from build123d import *

# Parameters (mm, degrees)
F0_W     = 231
F0_H     = 310
F1_DEPTH = 4
F2_W     = 310
F2_H     = 16
F3_DEPTH = 4


with BuildPart() as f1:
    # F0 (on Top) → F1 (new body)
    with BuildSketch(Plane.XY):
        with Locations((115.5, 155)):
            Rectangle(F0_W, F0_H)
    extrude(amount=F1_DEPTH)

    # F2 (on Right) → F3 (join)
    with BuildSketch(Plane.YZ):
        with Locations((155, 8)):
            Rectangle(F2_W, F2_H)
    extrude(amount=F3_DEPTH)

    # F4: F1 across face


with BuildPart() as f1_1:
    add(f1.part)
    add(f1.part.mirror(Plane(origin=(231, 155, 2), x_dir=(0, 1, 0), z_dir=(1, 0, 0))))

    # F5: F1 across face


with BuildPart() as f1_2:
    add(f1_1.part)
    add(f1_1.part.mirror(Plane(origin=(231, 0, 2.395062), x_dir=(1, 0, 0), z_dir=(0, -1, 0))))


solid = f1_2.part
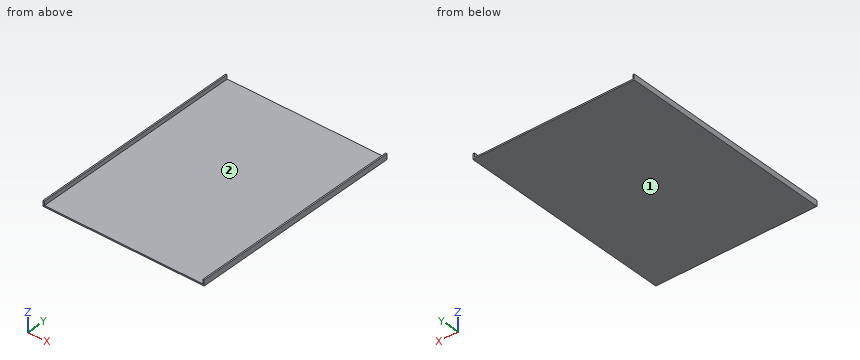
Input: part model. Units: mm. Frame: model coordinates. Face numbers are marked on the shaded views. Coordinates: 2 decimals unless noted, no trailing zeros. Loops run counter-clockwise (first coordinate to the right, second up) from the corner with the lowest first, then second, coordinate; pieces in that order, holes last. Notation, with made-up numbers: (-39.75, 68) -> (-5.75, 68) arc R9 ccw to (-5.75, 80) -> close; hole circle Ø7 at (-4, 17). An arc over 180 degrees is marked (long way). Write each question's results on one line, items separated by ' | '. Start each with the question number.
Q1. Section C-C, the plane x = 307. Return the cut outline in (y, z), plus the area to 3 significant figures.
Q2. Section B-B, the plane y = -42.5. Return the cut outline in (x, z), plus the area to 3 significant figures.
Q3. Pull-direction query (X, two-part tool) for the marked faces 1 and 2; classes: released by +X, released by -X, zero draft, split by the parting line, or undercut.
Q4. Section A-A, the plane z = 11. Return the cut outline in (x, y).
Q5. Ray query, line 1 (X direction, y = -243.5, z = 9.5); line 2 (Z direction, x = 177.5, y = 120). Return the intervals inside material, ascending. Write a range as from..to.
Found:
1) outline: (-310, 0) -> (310, 0) -> (310, 4) -> (-310, 4) -> close | area: 2,480 mm2
2) outline: (0, 0) -> (462, 0) -> (462, 16) -> (458, 16) -> (458, 4) -> (4, 4) -> (4, 16) -> (0, 16) -> close | area: 1,940 mm2
3) face 1: zero draft | face 2: undercut
4) outline: (0, -310) -> (4, -310) -> (4, 310) -> (0, 310) -> close; (458, -310) -> (462, -310) -> (462, 310) -> (458, 310) -> close
5) line 1: 0..4, 458..462 | line 2: 0..4
